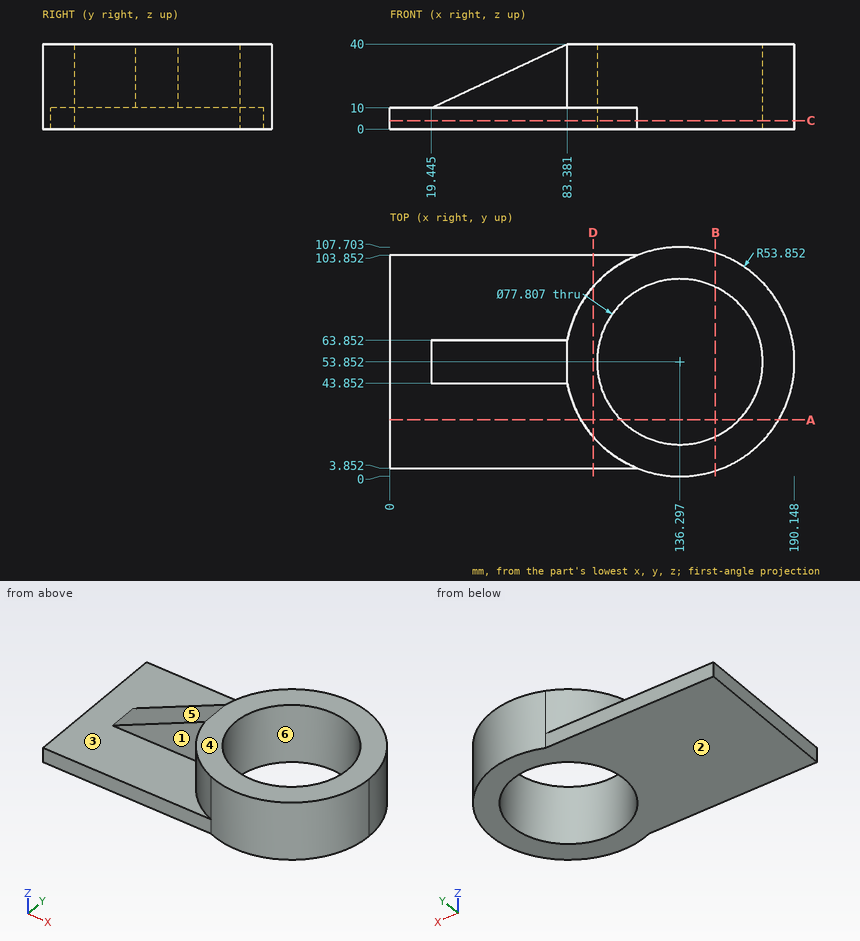
Geometry check sheet. Reference: drawing and pictorial views, mm from the part's lowest x, y, z. A direction names the side the tool comes from. Round coordinates to 2 decimals unless told otherwise and drop trailing zeros. Loops run counter-clockwise (first coordinate to the right, second up) from the corner with the lowest first, then second, coordinate; pieces in that order, holes last. Notation, with made-up numbers: (-29.5, 77) - (-7.5, 77) arc R25 cw to (-7.5, 97) - close; hole circle Ø1 at (85.5, -12). An arc over 180 degrees is marked (long way). Use a Markdown table: item, result.
Q1. Material ranges on line 1 (Z direction, x = 15, y = 12.5); line 2 (X direction, y = 46.5, z = 22) (1 decimal); line 3 (Y direction, x = 49.5, z = 14), recorded low to high.
Solutions:
| item | result |
|---|---|
| line 1 | z = 0 to 10 |
| line 2 | x = 45 to 98.1, 174.5 to 189.6 |
| line 3 | y = 43.85 to 63.85 |
Q2. Access from +Z, -Z, +X, -X, +Y, -Y to the whole of each face (thin tool, end or side, straight path). Record for the marked faces 1, 2 and 3.
Solutions:
| item | result |
|---|---|
| face 1 | +Z, -X, -Y |
| face 2 | -Z, +X, -X, +Y, -Y |
| face 3 | +Z, -X |
Q3. Cross-section at D-D on x = 95.5. Record the cut outline in (y, z), plus the area to 3 significant figures.
Solutions:
| item | result |
|---|---|
| outline | (3.85, 0) - (103.85, 0) - (103.85, 10) - (89, 10) - (89, 40) - (18.7, 40) - (18.7, 10) - (3.85, 10) - close |
| area | 3,110 mm2 |
Q4. Go/stop test with flat-tipped pins: P1, Ø1.5, axis at x = 50.5, z = 19, coming from the +Y side; P2, Ø2, axis at y = 45.5, z = 7, coming from the +X side; P3, Ø24, axis at x = 49, z = 19.5, coming from the -Y side. Record where each tip stops, or that it passes through.
Solutions:
| item | result |
|---|---|
| P1 | stops at y = 63.85 |
| P2 | stops at x = 189.64 |
| P3 | stops at y = 3.85 |
Q5. Cross-section at A-A on y = 26.5. Record the cut outline in (x, z) (1 decimal), plus the area to 3 significant figures.
Solutions:
| item | result |
|---|---|
| outline | (0, 0) - (108.6, 0) - (108.6, 40) - (89.9, 40) - (89.9, 10) - (0, 10) - close; (164, 0) - (182.7, 0) - (182.7, 40) - (164, 40) - close |
| area | 2,400 mm2 |
Q6. Draft check along X on the marked faces 4, 5 and 6. Enter one of: released by +X, released by -X, zero draft, split by the parting line, or undercut.
Solutions:
| item | result |
|---|---|
| face 4 | zero draft |
| face 5 | released by -X |
| face 6 | undercut |
Q7. Cross-section at B-B on x = 153. Record the cut outline in (y, z).
Solutions:
| item | result |
|---|---|
| outline | (2.66, 0) - (18.72, 0) - (18.72, 40) - (2.66, 40) - close; (88.99, 0) - (105.05, 0) - (105.05, 40) - (88.99, 40) - close |
Q8. Cross-section at C-C on z = 4. Record the cut outline in (x, y).
Solutions:
| item | result |
|---|---|
| outline | (0, 3.85) - (116.3, 3.85) arc R53.85 ccw to (190.15, 53.85) arc R53.85 ccw to (116.3, 103.85) - (0, 103.85) - close; hole circle Ø77.81 at (136.3, 53.85) |
